Here's how the part is built. I have some questions about the finished solid (model axes, mm). A direction names the side the tool comes from. Give positions to 0.01 mm unless a question says otherwise; leave off trailing zeros. Write each loop counter-clockwise with the first axis right and the second up, starting at its lowest first coordinate (ties: lowest second). Pieces come first, ordered by that corner, then holes. Notation, with made-up numbers: (-24.75, -10.5) - (8.25, -10.5) arc R20 cw to (8.25, 14.5) - close; hole circle Ø10 at (47.5, 22). An arc over 180 degrees is marked (long way). One line per item, written item: value. Start each with the question number.
1) Imagine slicing it at C-C on x = 45. Write out the boundary of the cut face in (y, z).
2) We'd pull the mould along X, two halves only. Please class faces 4 (the flat face through (25.262, 41, 0)), 5 (the cylindrical face through (31.891, 44.231, 1.102)), 6 (the cylindrical face through (49.82, 43.76, 0.95)), 7 (the flat face through (43.397, 43, -2)): +X half, -X half, draft (parallel to the pull), parting line (faces both ways), or undercut.
3) Please list where these lines run through material, in increasing order: L1, parallel to Z at x = 41.5, y = 40.75; L2, parallel to X at y = 39.5, z = 3; L3, parallel to Y at x = 30, z = -0.25. Write a range as [from, to].
4) On a 3-axis mill with a long thin cutter (end or side, diameter ignored), from which of +Z, -Z, +X, -X, +Y, -Y can I reach the whole of each face in a straight line? I mean faces 1 (the cylindrical face through (28.393, 35.288, 0.24)), 2 (the flat face through (30.697, 39, 4)), 3 (the flat face through (45.759, 38, 1)). Say none if no direction works.
5) I'm going to push flat-ended pins straight in: P1, Ø6, axis at x = 51, y = 45, coming from the -Z side; P2, Ø3, axis at x = 51.5, z = -3, coming from the +Y side; P3, Ø4, axis at x = 37.5, z = 0.5, coming from the -Y side. Where does each tip first touch, or does it pass through?
6) Imagine slicing it at B-B on x = 37.25. Write out the boundary of the cut face in (y, z), plus the area to 3 significant figures.
from build123d import *


with BuildPart() as part:
    # Sketch1 → Revolve1 (revolve)
    with BuildSketch(Plane.XY):
        with BuildLine():
            Line((26.023627587, 46.178938329), (30.697227587, 46.178938329))
            Line((30.697227587, 46.178938329), (30.697227587, 44.908938329))
            Line((30.697227587, 44.908938329), (30.697227587, 44.654938329))
            ThreePointArc((30.697227587, 44.654938329), (30.771622465, 44.475333206), (30.951227587, 44.400938329))
            Line((30.951227587, 44.400938329), (31.205227587, 44.400938329))
            Line((31.205227587, 44.400938329), (32.805427587, 44.400938329))
            ThreePointArc((32.805427587, 44.400938329), (32.98503271, 44.475333206), (33.059427587, 44.654938329))
            Line((33.059427587, 44.654938329), (43.397227587, 44.654938329))
            Line((43.397227587, 44.654938329), (43.397227587, 43.600838329))
            ThreePointArc((43.397227587, 43.600838329), (43.546017342, 43.241628084), (43.905227587, 43.092838329))
            Line((43.905227587, 43.092838329), (45.505427587, 43.092838329))
            ThreePointArc((45.505427587, 43.092838329), (45.68503271, 43.167233206), (45.759427587, 43.346838329))
            Line((45.759427587, 43.346838329), (45.759427587, 43.905638329))
            Line((45.759427587, 43.905638329), (53.760427587, 43.905638329))
            Line((53.760427587, 43.905638329), (54.522427587, 43.143638329))
            Line((54.522427587, 43.143638329), (54.522427587, 40.730638329))
            Line((54.522427587, 40.730638329), (25.261627587, 40.730638329))
            Line((25.261627587, 40.730638329), (25.261627587, 45.416938329))
            Line((25.261627587, 45.416938329), (26.023627587, 46.178938329))
        make_face()
    revolve(axis=Axis((25.261627587, 40.730638329, 0), (1, 0, 0)))


solid = part.part
Numbers:
1. outline: circle Ø4.72 at (40.73, 0)
2. face 4: -X half
2. face 5: undercut
2. face 6: draft
2. face 7: undercut
3. L1: [-3.92, 3.92]
3. L2: [25.26, 43.4]
3. L3: [35.29, 46.17]
4. face 1: +X, -X
4. face 2: +X
4. face 3: none
5. P1: z = -2.91
5. P2: y = 43.53
5. P3: y = 36.81
6. outline: circle Ø7.85 at (40.73, 0)
6. area: 48.4 mm^2
